from build123d import *

# Parameters (mm, degrees)
BOSS_EXTRUDE1_DEPTH = 18.8
SKETCH2_W           = 3.45
SKETCH2_H           = 20.125
CUT_EXTRUDE1_DEPTH  = 73.204371405
CUT_EXTRUDE2_REACH  = 45.006
SKETCH3_R           = 1.5
BOSS_EXTRUDE2_REACH = 44.46
SKETCH7_W           = 3.75
SKETCH7_H           = 4
CUT_EXTRUDE8_DEPTH  = 2.5


with BuildPart() as part:
    # Sketch1 → Boss-Extrude1 (new body)
    with BuildSketch(Plane(origin=(0, 0, 0), x_dir=(0, 0, -1), z_dir=(1, 0, 0))):
        Polygon((-25.0625, 0), (25.0625, 0), (25.0625, -20.875), (32.5625, -20.875), (32.5625, -24.875), (25.0625, -24.875), (20.0625, -24.875), (20.0625, -5), (-20.0625, -5), (-20.0625, -24.875), (-25.0625, -24.875), (-32.5625, -24.875), (-32.5625, -20.875), (-25.0625, -20.875), align=None)
    extrude(amount=BOSS_EXTRUDE1_DEPTH)

    # Sketch2 → Cut-Extrude1 (cut, through all)
    with BuildSketch(Plane.XY.offset(32.5625)):
        with Locations((9.4, -14.8125)):
            Rectangle(SKETCH2_W, SKETCH2_H)
    extrude(amount=-CUT_EXTRUDE1_DEPTH, mode=Mode.SUBTRACT)

    # Sketch3 → Cut-Extrude2 (cut, up to next)
    with BuildSketch(Plane(origin=(0, -20.875, 0), x_dir=(1, 0, 0), z_dir=(0, 1, 0)), mode=Mode.PRIVATE) as cut_extrude2_sk1:
        with Locations(Location((3.8375, -28.8125, 0), (0, 0, 270))):
            Circle(SKETCH3_R)
    cut_extrude2_tool1 = extrude(cut_extrude2_sk1.sketch, amount=-CUT_EXTRUDE2_REACH, mode=Mode.PRIVATE) & part.part
    # Sketch3 → Cut-Extrude2 (cut, up to next)
    with BuildSketch(Plane(origin=(0, -20.875, 0), x_dir=(1, 0, 0), z_dir=(0, 1, 0)), mode=Mode.PRIVATE) as cut_extrude2_sk2:
        with Locations(Location((14.9625, -28.8125, 0), (0, 0, 270))):
            Circle(SKETCH3_R)
    cut_extrude2_tool2 = extrude(cut_extrude2_sk2.sketch, amount=-CUT_EXTRUDE2_REACH, mode=Mode.PRIVATE) & part.part
    # Sketch3 → Cut-Extrude2 (cut, up to next)
    with BuildSketch(Plane(origin=(0, -20.875, 0), x_dir=(1, 0, 0), z_dir=(0, 1, 0)), mode=Mode.PRIVATE) as cut_extrude2_sk3:
        with Locations(Location((14.9625, 28.8125, 0), (0, 0, 270))):
            Circle(SKETCH3_R)
    cut_extrude2_tool3 = extrude(cut_extrude2_sk3.sketch, amount=-CUT_EXTRUDE2_REACH, mode=Mode.PRIVATE) & part.part
    # Sketch3 → Cut-Extrude2 (cut, up to next)
    with BuildSketch(Plane(origin=(0, -20.875, 0), x_dir=(1, 0, 0), z_dir=(0, 1, 0)), mode=Mode.PRIVATE) as cut_extrude2_sk4:
        with Locations(Location((3.8375, 28.8125, 0), (0, 0, 270))):
            Circle(SKETCH3_R)
    cut_extrude2_tool4 = extrude(cut_extrude2_sk4.sketch, amount=-CUT_EXTRUDE2_REACH, mode=Mode.PRIVATE) & part.part
    add(cut_extrude2_tool1.solids().sort_by_distance((3.8375, -20.875, 28.8125))[0], mode=Mode.SUBTRACT)
    add(cut_extrude2_tool2.solids().sort_by_distance((14.9625, -20.875, 28.8125))[0], mode=Mode.SUBTRACT)
    add(cut_extrude2_tool3.solids().sort_by_distance((14.9625, -20.875, -28.8125))[0], mode=Mode.SUBTRACT)
    add(cut_extrude2_tool4.solids().sort_by_distance((3.8375, -20.875, -28.8125))[0], mode=Mode.SUBTRACT)

    # Sketch7 → Boss-Extrude2 (add, up to next)
    with BuildSketch(Plane(origin=(7.675, 0, 0), x_dir=(0, 0, -1), z_dir=(1, 0, 0)), mode=Mode.PRIVATE) as boss_extrude2_sk1:
        with Locations((-30.6875, -22.875)):
            Rectangle(SKETCH7_W, SKETCH7_H)
    boss_extrude2_tool1 = extrude(boss_extrude2_sk1.sketch, amount=BOSS_EXTRUDE2_REACH, mode=Mode.PRIVATE) - part.part
    boss_extrude2 = boss_extrude2_tool1.solids().sort_by_distance((7.675, -22.875, 30.6875))[0]
    add(boss_extrude2)

    # Mirror1: Boss-Extrude2 across plane
    add(boss_extrude2.mirror(Plane.XY))

    # Sketch4 → Cut-Extrude8 (cut)
    with BuildSketch(Plane(origin=(7.675, 0, 0), x_dir=(0, 0, -1), z_dir=(1, 0, 0))):
        Polygon((-20.0625, -24.875), (-20.0625, -15.75), (-20.0625, -14), (-25.0625, -14), (-25.0625, -15.75), (-25.0625, -24.875), align=None)
    extrude(amount=-CUT_EXTRUDE8_DEPTH, mode=Mode.SUBTRACT)


solid = part.part
Geometry: final body of the model. Coordinates: model frame, mm. A direction names the side the tool comes from. Coordinates: 2 decimals unless noted, no trailing zeros. Write each loop counter-clockwise with the first axis right and the second up, starting at its lowest first coordinate (ties: lowest second). Pieces come first, ordered by that corner, then holes. Notation, with made-up numbers: (5.25, 40) - (25.25, 40) arc R12 cw to (25.25, 49) - close; hole circle Ø1 at (42.25, 43). An arc over 180 degrees is marked (long way). Return JSON: item names as keys, results as strings.
Item 1: Section query C-C (z = -26). Output: boundary loops of the cut face in (x, y) (3 decimals), and give its area (3 significant figures).
Completed:
{"outline": "(0, -24.875) - (7.675, -24.875) - (7.675, -20.875) - (0, -20.875) - close; (11.125, -24.875) - (18.8, -24.875) - (18.8, -20.875) - (11.125, -20.875) - close", "area": "61.4 mm2"}
Item 2: Pull-direction query (Z, two-part tool) for faces 1 (the face through (3.903, -22.847, 27.314)), 2 (the face through (11.4, -24.875, 26.4)), 3 (the face through (9, -23, 32.562)), 4 (the face through (6, -23, 25.062)); classes: +Z half, -Z half, draft (parallel to the pull), parting line (faces both ways), or undercut.
Completed:
{"face 1": "undercut", "face 2": "draft", "face 3": "+Z half", "face 4": "undercut"}
Item 3: Line query: L1, parallel to Z at x = 4, y = -20.5; L2, parallel to X at y = -23.5, z = -27 (3 decimals); L3, parallel to Z at x = 9.75, y = -22.25. Output: solid intervals per line, ascending.
Completed:
{"L1": "z = -25.06 to -20.06, 20.06 to 25.06", "L2": "x = 0 to 7.675, 11.125 to 18.8", "L3": "z = -32.56 to -28.81, 28.81 to 32.56"}
Item 4: Section query D-D (z = 4). Output: boundary loops of the cut face in (x, y) (3 decimals).
Completed:
{"outline": "(0, -5) - (7.675, -5) - (7.675, -4.75) - (11.125, -4.75) - (11.125, -5) - (18.8, -5) - (18.8, 0) - (0, 0) - close"}
Item 5: Reachability of faces 5 (the face through (9, -4.75, 0)), 6 (the face through (7.675, -13, -22)), 7 (the face through (11.4, -10.6, 25.062)), 8 (the face through (15, -5, 0)) from +Z, -Z, +X, -X, +Y, -Y: full face, straight path, thin tool, end or side. Return the list, or none.
Completed:
{"face 5": "+Z, -Z, -Y", "face 6": "-Y", "face 7": "+Z, +X, -X, +Y", "face 8": "+X, -X, -Y"}
Item 6: Section query A-A (x = 10.5). Count the separate pieces of the cut face and the enclosed holes in it, and give its area (3 significant figures).
Completed:
{"separate pieces": "3", "enclosed holes": "0", "area": "268 mm2"}
Item 7: Section query B-B (y = -16). Output: boundary loops of the cut face in (x, z) (1 decimal).
Completed:
{"outline": "(0, -25.1) - (7.7, -25.1) - (7.7, -20.1) - (0, -20.1) - close; (0, 20.1) - (5.2, 20.1) - (5.2, 25.1) - (0, 25.1) - close; (11.1, -25.1) - (18.8, -25.1) - (18.8, -20.1) - (11.1, -20.1) - close; (11.1, 20.1) - (18.8, 20.1) - (18.8, 25.1) - (11.1, 25.1) - close"}
Item 8: Pin query (flat end, axial travel): pin 1 Ø10 at (x, y) = (7, -14) entering from -Z; pin 2 Ø2.5 at (x, z) = (4.5, 8) entering from -Y; pin 3 Ø0.8 at (x, z) = (7, 23) entering from -Y. Return the tip coordinate at first contact, or that it passes through.
Completed:
{"pin 1": "stops at z = -25.06", "pin 2": "stops at y = -5", "pin 3": "stops at y = -14"}
